Here's how the part is built. I have some questions about the finished solid (model axes, mm). A direction names the side the tool comes from. Coordinates: 2 decimals unless noted, no trailing zeros. Order: outer loops, then holes, each group sorted by start corner. A loop starts at its lowest first (then second) coordinate and runs counter-clockwise, first axis right, second up. Notation, with made-up numbers: (47, 62.5) - (102, 62.5) arc R24 cw to (102, 73.5) - close; hole circle Ø1 at (37.25, 89). An arc over 180 degrees is marked (long way). Answer as CSV lines item,"result". Start each with the question number.
Q1. Suppose I cut it at B-B (x = 17.5). Please give me the cut outline in (y, z).
Q2. Suppose I cut it at A-A (x = -2). Please give me the cut outline in (y, z).
Q3. For faces 1 (the face through (6.342, 6, -6)), 2 (the face through (10.99, 68.03, 7.15)), 3 (the face through (6.342, 17, 4)), 4 (the face through (38.37, 39.75, 5.06)), which set-ups out of +Z, -Z, +X, -X, +Y, -Y let a thin tool reach every point of the face, with its end or its side?
Q4. For pin 1 Ø7.5 at (x, z) = (25.5, -4) entering from -Y; pin 2 Ø1.5 at (y, z) = (66.5, -4.5) entering from -X; pin 3 Ø2.5 at (x, z) = (21, 5) entering from +Y; pin 4 Ø1.5 at (x, y) = (43, -5) entering from -Z, each with a flat end and sliding along its axis, tell me the tip position at first contact or that it passes through.
Q5. Thinking about a two-plate mould opening in Y: for faces 5 (the face through (11.081, 93.524, -12.346)), 6 (the face through (30, 7.323, -3)), 7 (the face through (49, 2.328, 5)), which applies, released by +Y, released by -Y, zero draft, split by the parting line, or undercut?
Q6. Suppose I cut it at D-D (z = -10.5). Count the separate pieces of the cut face and the enclosed holes in it, then the cut area to 3 significant figures.
Q7. I need wall thicknesses on line 1 (Y direction, x = 36, z = -4); line 2 (Z direction, x = 55, y = 7); line 3 (Z direction, x = 11, y = 15). Which ranges of each line are inside material? Lowest first, please.
Q8. Suppose I cut it at C-C (y = 9.5). Please give me the cut outline in (x, z), then the cut area to 3 significant figures.
from build123d import *

# Parameters (mm, degrees)
SKETCH2_R           = 1.7500000000000018
SKETCH2_R_2         = 1.7499999999999967
SKETCH2_R_3         = 1.7500000000000013
SKETCH2_R_4         = 1.7500000000000038
BOSS_EXTRUDE2_DEPTH = 5
SKETCH5_W           = 31.39999999999999
SKETCH5_H           = 2.3000000000000007
BOSS_EXTRUDE4_DEPTH = 10
CUT_EXTRUDE1_DEPTH  = 77.48529270389177
FILLET1_RADIUS      = 10
FILLET1_LENGTH      = 5
SKETCH7_W           = 31.39999999999999
SKETCH7_H           = 13.340000000000003
CUT_EXTRUDE3_DEPTH  = 4
SKETCH8_W           = 8
SKETCH8_H           = 28
BOSS_EXTRUDE5_DEPTH = 32
BOSS_EXTRUDE6_DEPTH = 8
SKETCH10_R          = 2.500000000000001
CUT_EXTRUDE4_DEPTH  = 92.61877536837086
CUT_EXTRUDE5_DEPTH  = 89.05679985100527
FILLET3_R           = 4
FILLET2_R           = 4
FILLET4_R           = 4
SCALE1_SCALE        = 1.5


with BuildPart() as part:
    # Sketch2 → Boss-Extrude2 (new body)
    with BuildSketch(Plane.XY):
        Polygon((25.999999999999996, 45), (9.999999999999998, 45), (0, 33.819660112501055), (0, 15.000000000000002), (10.000000000000002, 0), (26, 0), (36.00000000000001, 14.999999999999993), (60, 14.999999999999996), (60, 35), (36.00000000000001, 35), align=None)
        with Locations((12.999999999999998, 5.000000000000004)):
            Circle(SKETCH2_R, mode=Mode.SUBTRACT)
        with Locations((22.999999999999993, 5.000000000000004)):
            Circle(SKETCH2_R_2, mode=Mode.SUBTRACT)
        with Locations((5.000000000000001, 24.999999999999993)):
            Circle(SKETCH2_R_3, mode=Mode.SUBTRACT)
        with Locations((32.129999999999995, 24.999999999999993)):
            Circle(SKETCH2_R_4, mode=Mode.SUBTRACT)
    extrude(amount=BOSS_EXTRUDE2_DEPTH)

    # Sketch5 → Boss-Extrude4 (add)
    with BuildSketch(Plane(origin=(0, 0, 0), x_dir=(-1, 0, 0), z_dir=(0, 0, -1))):
        with Locations((-25.4, 17.179999999999993)):
            Rectangle(SKETCH5_W, SKETCH5_H)
        with Locations((-25.4, 32.82)):
            Rectangle(SKETCH5_W, SKETCH5_H)
    extrude(amount=BOSS_EXTRUDE4_DEPTH)

    # Sketch6 → Cut-Extrude1 (cut, through all)
    with BuildSketch(Plane.XY.offset(5)):
        Polygon((60, 35), (49.999999999999986, 35), (49.99999999999999, 14.999999999999993), (60, 14.999999999999993), align=None)
    extrude(amount=-CUT_EXTRUDE1_DEPTH, mode=Mode.SUBTRACT)

    # Fillet1: full round fillet: the end face becomes a half cylinder, R = half its width
    fillet1_face = Plane((50, 25, 2.5), x_dir=(0, 0, -1), z_dir=(1, 0, 0))  # on the end face: x along it, z out of the body
    fillet1_slab = fillet1_face.offset(-FILLET1_RADIUS / 2) * Box(FILLET1_LENGTH, 2 * FILLET1_RADIUS, FILLET1_RADIUS, mode=Mode.PRIVATE)  # the body's end, R deep
    fillet1_round = Plane((40, 25, 2.5), x_dir=(1, 0, 0), z_dir=(0, 0, -1)) * Cylinder(FILLET1_RADIUS, FILLET1_LENGTH, mode=Mode.PRIVATE)  # its axis R under the face
    add(fillet1_slab - fillet1_round, mode=Mode.SUBTRACT)

    # Sketch7 → Cut-Extrude3 (cut)
    with BuildSketch(Plane(origin=(0, 0, 0), x_dir=(-1, 0, 0), z_dir=(0, 0, -1))):
        with Locations((-25.4, 24.999999999999996)):
            Rectangle(SKETCH7_W, SKETCH7_H)
    extrude(amount=-CUT_EXTRUDE3_DEPTH, mode=Mode.SUBTRACT)

    # Sketch8 → Boss-Extrude5 (add)
    with BuildSketch(Plane(origin=(0, 45, 0), x_dir=(1, 0, 0), z_dir=(0, 1, 0))):
        with Locations((9.999999999999996, 9)):
            Rectangle(SKETCH8_W, SKETCH8_H)
    extrude(amount=BOSS_EXTRUDE5_DEPTH)

    # Sketch9 → Boss-Extrude6 (add)
    with BuildSketch(Plane.ZY.offset(-5.999999999999995)):
        Polygon((5.000000000000001, 45), (-23, 45), (-15.299548194431079, 39.40983005625053), (5, 39.40983005625053), align=None)
    extrude(amount=-BOSS_EXTRUDE6_DEPTH)

    # Sketch10 → Cut-Extrude4 (cut, through all)
    with BuildSketch(Plane.ZY.offset(-5.999999999999995)):
        with Locations((-9, 63)):
            Circle(SKETCH10_R)
    extrude(amount=-CUT_EXTRUDE4_DEPTH, mode=Mode.SUBTRACT)

    # Sketch11 → Cut-Extrude5 (cut, through all)
    with BuildSketch(Plane(origin=(13.999999999999995, 0, 0), x_dir=(0, 0, -1), z_dir=(1, 0, 0))):
        Polygon((0, 39.40983005625053), (23, 57.30500139086019), (23, 45), (15.299548194431079, 39.40983005625053), align=None)
    extrude(amount=-CUT_EXTRUDE5_DEPTH, mode=Mode.SUBTRACT)

    # Fillet3
    fillet3_edges = [part.edges().sort_by_distance(p)[0] for p in [
        (9.999999999999995, 77, -23),
        (9.999999999999995, 77, 5.000000000000001),
        (9.999999999999995, 39.40983005625053, 0),
        (9.999999999999995, 57.30500139086019, -23),
    ]]
    fillet(fillet3_edges, radius=FILLET3_R)

    # Fillet2
    # the kernel refuses this fillet: 4 mm, written as the material it takes off along each edge
    with BuildSketch(Plane(origin=(13.999999999999995, 40.61090749308988, -1.5437002826498933), x_dir=(-1, 1.3e-16, 1e-16), z_dir=(0, 0.6140749293375269, -0.7892477311713423))) as fillet2_piece_1_section:
        with BuildLine():
            CenterArc((FILLET2_R, FILLET2_R), FILLET2_R, 180, 90)
            Line((6.8e-16, FILLET2_R), (0, 0))
            Line((0, 0), (FILLET2_R, 0))
        make_face()
    fillet2_piece_1 = extrude(amount=25.229846914032212, mode=Mode.PRIVATE)
    fillet2_piece_1 = split(fillet2_piece_1, bisect_by=Plane(origin=(13.08677452715668, 48.37488686948177, 0), z_dir=(0, 0, -1)), keep=Keep.TOP, mode=Mode.PRIVATE)
    add(fillet2_piece_1, mode=Mode.SUBTRACT)
    with BuildSketch(Plane(origin=(13.999999999999995, 59.26091487870621, -23), x_dir=(-1, 0, 0), z_dir=(0, 1, 0))) as fillet2_piece_2:
        with BuildLine():
            CenterArc((FILLET2_R, FILLET2_R), FILLET2_R, 180, 90)
            Line((0, FILLET2_R), (0, 0))
            Line((0, 0), (FILLET2_R, 0))
        make_face()
    extrude(amount=13.73908512129379, mode=Mode.SUBTRACT)
    with BuildSketch(Plane(origin=(13.999999999999995, 77, -19), x_dir=(-1, 0, 0), z_dir=(0, 0, 1))) as fillet2_piece_3:
        with BuildLine():
            CenterArc((FILLET2_R, FILLET2_R), FILLET2_R, 180, 90)
            Line((0, FILLET2_R), (0, 0))
            Line((0, 0), (FILLET2_R, 0))
        make_face()
    extrude(amount=20, mode=Mode.SUBTRACT)
    with BuildSketch(Plane(origin=(13.999999999999995, 45, 5.000000000000001), x_dir=(-1, 0, -2.2e-16), z_dir=(0, 1, 0))) as fillet2_piece_4:
        with BuildLine():
            CenterArc((FILLET2_R, -FILLET2_R), FILLET2_R, 90.00000000000001, 89.99999999999999)
            Line((2.66e-15, -FILLET2_R), (0, 0))
            Line((0, 0), (FILLET2_R, 0))
        make_face()
    extrude(amount=28, mode=Mode.SUBTRACT)
    with BuildSketch(Plane(origin=(13.999999999999995, 73, 1.0000000000000009), x_dir=(0, 0, 1), z_dir=(0, -1, 0))) as fillet2_piece_5:
        with BuildLine():
            CenterArc((4 - FILLET2_R, FILLET2_R), FILLET2_R, 270, 90)
            Line((4 - FILLET2_R, 0), (4, 0))
            Line((4, 0), (4, FILLET2_R))
        make_face()
    revolve(axis=Axis((13.999999999999995, 73, 1.0000000000000009), (-1, 0, 0)), revolution_arc=90, mode=Mode.SUBTRACT)
    with BuildSketch(Plane(origin=(13.999999999999995, 73, -19), x_dir=(0, 0, -1), z_dir=(0, -1, 0))) as fillet2_piece_6:
        with BuildLine():
            CenterArc((4 - FILLET2_R, -FILLET2_R), FILLET2_R, 0, 90)
            Line((4 - FILLET2_R, 0), (4, 0))
            Line((4, 0), (4, -FILLET2_R))
        make_face()
    revolve(axis=Axis((13.999999999999995, 73, -19), (1, 0, 0)), revolution_arc=90, mode=Mode.SUBTRACT)
    with BuildSketch(Plane(origin=(13.999999999999995, 59.26091487870621, -19), x_dir=(0, 0, -1), z_dir=(0, 1, 0))) as fillet2_piece_7:
        with BuildLine():
            CenterArc((4 - FILLET2_R, FILLET2_R), FILLET2_R, 270, 90)
            Line((4 - FILLET2_R, 0), (4, 0))
            Line((4, 0), (4, FILLET2_R))
        make_face()
    revolve(axis=Axis((13.999999999999995, 59.26091487870621, -19), (-1, 0, 0)), revolution_arc=52.11526627923318, mode=Mode.SUBTRACT)
    with BuildSketch(Plane(origin=(13.999999999999995, 37.453916568404516, -4.000000000000001), x_dir=(0, 0.7892477311713422, 0.614074929337527), z_dir=(0, 0.614074929337527, -0.7892477311713422))) as fillet2_piece_8_section:
        with BuildLine():
            CenterArc((3.999999999999998 + FILLET2_R, -FILLET2_R), FILLET2_R, 90.00000000000004, 89.99999999999994)
            Line((3.999999999999998 + FILLET2_R, 0), (3.999999999999998, 0))
            Line((3.999999999999998, 0), (4, -FILLET2_R))
        make_face()
    fillet2_piece_8 = revolve(axis=Axis((13.999999999999995, 37.453916568404516, -4.000000000000001), (1, 0, 0)), revolution_arc=195.37400527524528, mode=Mode.PRIVATE)
    fillet2_piece_8 = split(fillet2_piece_8, bisect_by=Plane(origin=(12.442859007716585, 39.2454758765285, 0), z_dir=(0, 0, -1)), keep=Keep.TOP, mode=Mode.PRIVATE)
    fillet2_piece_8 = split(fillet2_piece_8, bisect_by=Plane(origin=(12.442859007716585, 33.97, -0.3361174942439581), z_dir=(0, 1, 0)), keep=Keep.TOP, mode=Mode.PRIVATE)
    add(fillet2_piece_8, mode=Mode.SUBTRACT)

    # Fillet4
    fillet4_edges = [part.edges().sort_by_distance(p)[0] for p in [
        (5.999999999999995, 40.52786404500041, 2.500000000000001),
        (26, 0, 2.5),
        (10.000000000000002, 0, 2.5),
        (0, 15.000000000000002, 2.5),
        (0, 33.819660112501055, 2.5),
        (25.999999999999996, 45, 2.5),
        (36.00000000000001, 35, 2.5),
    ]]
    fillet(fillet4_edges, radius=FILLET4_R)


with BuildPart() as part_1:
    # Scale1: scaled about (16.416357699, 40.343462641, -2.727678487)
    add(part.part.scale(SCALE1_SCALE).moved(Location((-8.2081788495, -20.1717313205, 1.3638392435))))


solid = part_1.part
Here are the results:
1,outline,"(-20.17, 1.36) - (3.87, 1.36) - (3.87, -13.64) - (7.32, -13.64) - (7.32, 7.36) - (27.33, 7.36) - (27.33, -13.64) - (30.78, -13.64) - (30.78, 1.36) - (47.33, 1.36) - (47.33, 8.86) - (-20.17, 8.86) - close"
2,outline,"(-6.98, 1.36) - (15.04, 1.36) - (15.04, 8.86) - (-6.98, 8.86) - close; (19.61, 1.36) - (37.5, 1.36) - (37.5, 8.86) - (19.61, 8.86) - close"
3,face 1,"-Z, -X, -Y"
3,face 2,"+Z, +X, +Y"
3,face 3,"-Z"
3,face 4,"+Z, -Z, +X, +Y"
4,pin 1,"stops at y = 3.87"
4,pin 2,"stops at x = 0.79"
4,pin 3,"stops at y = 47.33"
4,pin 4,"passes through"
5,face 5,"released by +Y"
5,face 6,"undercut"
5,face 7,"released by -Y"
6,separate pieces,"4"
6,enclosed holes,"0"
6,area,"792 mm²"
7,line 1,"y = 3.87 to 7.32, 27.33 to 30.78"
7,line 2,"z = 1.36 to 8.86"
7,line 3,"z = 7.36 to 8.86"
8,outline,"(-8.21, 1.36) - (6.34, 1.36) - (6.34, 7.36) - (53.44, 7.36) - (53.44, 1.36) - (64.59, 1.36) - (64.59, 8.86) - (-8.21, 8.86) - close"
8,area,"263 mm²"
